Design review of the part built by this model. Coordinates are the model's own, in mm. Face numbers are marked on the shaded views. Coordinates: 2 decimals unless noted, no trailing zeros. Order: outer loops, then holes, each group sorted by start corner. A loop starts at its lowest first (then second) coordinate and runs counter-clockwise, first axis right, second up. Notation, with made-up numbers: M -21.75,22.5 L 23.25,22.5 A19 cw 23.25,37.5 Z; hole C 78,41 d9. An arc over 180 degrees is marked long. Answer as a JSON object with one key per item and string values.
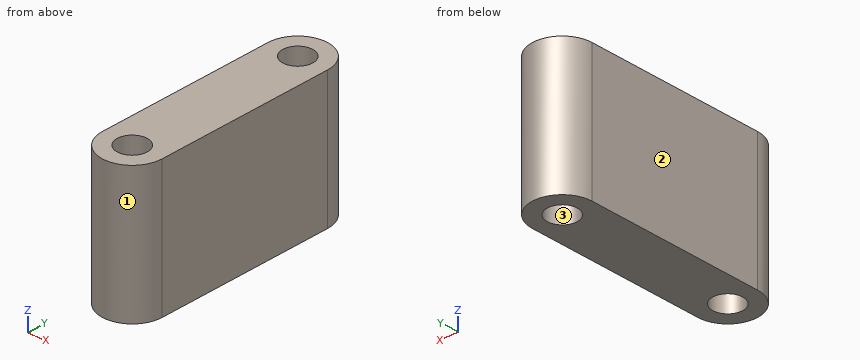
Autodesk Inventor part; units mm, degrees
ref_plane "YZ Plane" through (0, 0, 0) normal (1, 0, 0) x (0, 1, 0)
ref_plane "XZ Plane" through (0, 0, 0) normal (0, 1, 0) x (-1, 0, 0)
ref_plane "XY Plane" through (0, 0, 0) normal (0, 0, 1) x (1, 0, 0)
sketch "Sketch1" plane through (0, 0, 0) normal (0, 0, 1) x (1, 0, 0)
  line L0 (0, 0) -> (0, -19.05) construction
  line L1 (-3.175, 0) -> (-3.175, -19.05)
  line L2 (3.175, -19.05) -> (3.175, 0)
  arc A0 (3.175, 0) -> (-3.175, 0) centre (0, 0) ccw
  arc A1 (-3.175, -19.05) -> (3.175, -19.05) centre (0, -19.05) ccw
  circle A2 centre (0, 0) radius 1.5875
  circle A3 centre (0, -19.05) radius 1.5875
  point P0 (0, -9.525)
  dimension "d0" = 19.05
  dimension "d1" = 6.35
  dimension "d2" = 3.175
  dimension "d3" = 3.175
extrude "Extrusion1" add sketch "Sketch1" along normal blind 14.2875
properties part number "Bracket - 1" material "UHMW, White"
1) Add section A-A (x = 0). State the section outline as (y, z) points (1 decimal).
Taken from the geometry:
{"outline": "M -22.2,0 L -20.6,0 L -20.6,14.3 L -22.2,14.3 Z; M -17.5,0 L -1.6,0 L -1.6,14.3 L -17.5,14.3 Z; M 1.6,0 L 3.2,0 L 3.2,14.3 L 1.6,14.3 Z"}
2) Add section B-B (z = 9.25). Count the separate pieces of the cut face and the enclosed holes in it, and give its area (3 significant figures).
Taken from the geometry:
{"separate pieces": "1", "enclosed holes": "2", "area": "137 mm2"}
3) Add section C-C (y = -19.75). State the section outline as (x, z) points.
Taken from the geometry:
{"outline": "M -3.1,0 L -1.42,0 L -1.42,14.29 L -3.1,14.29 Z; M 1.42,0 L 3.1,0 L 3.1,14.29 L 1.42,14.29 Z"}
4) To check wall thickness, follow L1, parallel to Y at x = 0, z = 4.25 (1 decimal); L2, parallel to Y at x = -0.75, z = 7.5; L3, parallel to Y at x = 1.75, z = 11.5. State the ranges of each line that lie inside material, in increasing order.
Taken from the geometry:
{"L1": "y = -22.2 to -20.6, -17.5 to -1.6, 1.6 to 3.2", "L2": "y = -22.14 to -20.45, -17.65 to -1.4, 1.4 to 3.09", "L3": "y = -21.7 to 2.65"}
5) Mouldability with a two-part tool opening along X and no side actions: class the marked faces 1, 2 and 3 as released by +X, released by -X, zero draft, split by the parting line, or undercut.
Taken from the geometry:
{"face 1": "split by the parting line", "face 2": "released by -X", "face 3": "undercut"}
6) Insertion check: pin 1 Ø1 at (x, z) = (1.5, 1.5) entering from +Y; pin 2 Ø1 at (x, z) = (1, 12) entering from -Y; pin 3 Ø1.9 at (x, y) = (0, -19.05) entering from +Z. Each pin has a flat end and moves straight along its axis. Give the tip position at first contact, or say it passes through.
Taken from the geometry:
{"pin 1": "stops at y = 3.01", "pin 2": "stops at y = -22.19", "pin 3": "passes through"}
7) Add section D-D (y = 1.25). State the section outline as (x, z) points, and give its area (3 significant figures).
Taken from the geometry:
{"outline": "M -2.92,0 L -0.98,0 L -0.98,14.29 L -2.92,14.29 Z; M 0.98,0 L 2.92,0 L 2.92,14.29 L 0.98,14.29 Z", "area": "55.4 mm2"}
